For this review, take the finished solid that the model builds, in its own axes (mm). Face numbers are marked on the shaded views. A direction names the side the tool comes from. Round coordinates to 2 decimals unless told otherwise and drop trailing zeros. Write each loop counter-clockwise with the first axis right and the second up, starting at its lowest first coordinate (ties: lowest second). Pieces come first, ordered by that corner, then holes. Notation, with made-up numbers: (66.25, 49) -> (80.25, 49) arc R12 ccw to (80.25, 59) -> close; hole circle Ø11 at (-8.75, 61). An arc over 180 degrees is marked (long way). Answer in a Markdown table with one row per item.
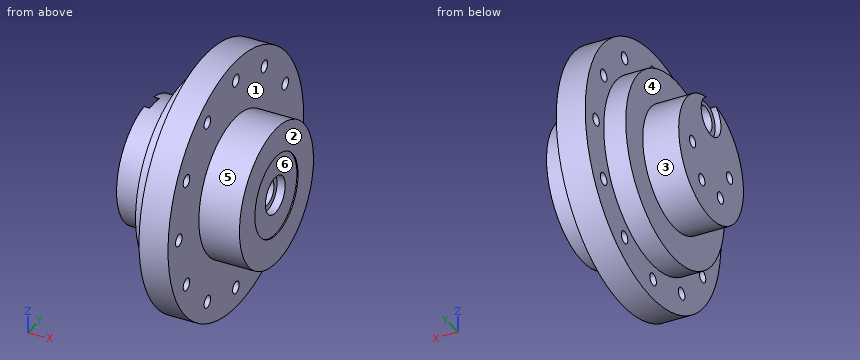
from build123d import *

# Parameters (mm, degrees)
SKETCH2_R          = 35
CUT_EXTRUDE1_DEPTH = 1
CUT_EXTRUDE2_REACH = 174.699
SKETCH3_R          = 5.25
CIRPATTERN1_COUNT  = 12
SKETCH9_R          = 5
CUT_EXTRUDE3_DEPTH = 10
CIRPATTERN2_COUNT  = 4
CIRPATTERN2_ANGLE  = 180


with BuildPart() as part:
    # Sketch1 → Revolve1 (revolve)
    with BuildSketch(Plane.XY, mode=Mode.PRIVATE) as revolve1_sk:
        Polygon((-290.135135135, 60), (-325.135135135, 60), (-325.135135135, 110), (-350.135135135, 110), (-350.135135135, 80), (-369.135135135, 80), (-369.135135135, 52.5), (-400.135135135, 52.5), (-400.135135135, 0), (-290.135135135, 0), align=None)
    revolve(revolve1_sk.sketch.rotate(Axis((-400.135135135, 0, 0), (1, 0, 0)), 90), axis=Axis((-400.135135135, 0, 0), (1, 0, 0)))

    # Sketch2 → Cut-Extrude1 (cut)
    with BuildSketch(Plane(origin=(-290.135135135, 0, 0), x_dir=(0, 0, -1), z_dir=(1, 0, 0))):
        Circle(SKETCH2_R)
    extrude(amount=-CUT_EXTRUDE1_DEPTH, mode=Mode.SUBTRACT)

    # Sketch3 → Cut-Extrude2 (cut, up to next)
    with BuildSketch(Plane(origin=(-325.135135135, 0, 0), x_dir=(0, 0, -1), z_dir=(1, 0, 0)), mode=Mode.PRIVATE) as cut_extrude2_sk1:
        with Locations((0, 92.5)):
            Circle(SKETCH3_R)
    cut_extrude2_tool1 = extrude(cut_extrude2_sk1.sketch, amount=-CUT_EXTRUDE2_REACH, mode=Mode.PRIVATE) & part.part
    cut_extrude2 = cut_extrude2_tool1.solids().sort_by_distance((-325.135135, 92.5, 0))[0]
    add(cut_extrude2, mode=Mode.SUBTRACT)

    # CirPattern1: Cut-Extrude2 ×12 about axis
    cirpattern1_axis = Axis((0, 0, 0), (1, 0, 0))
    for i in range(1, CIRPATTERN1_COUNT):
        add(cut_extrude2.rotate(cirpattern1_axis, i * 360 / CIRPATTERN1_COUNT), mode=Mode.SUBTRACT)

    # Sketch4 → Cut-Revolve1 (revolve, cut)
    with BuildSketch(Plane.XY, mode=Mode.PRIVATE) as cut_revolve1_sk:
        Polygon((-291.135135135, 16), (-298.135135135, 16), (-298.135135135, 11), (-328.635135135, 11), (-328.635135135, 17), (-353.635135135, 17), (-353.635135135, 11), (-374.135135135, 11), (-374.135135135, 16), (-381.135135135, 16), (-381.135135135, 0), (-291.135135135, 0), align=None)
    revolve(cut_revolve1_sk.sketch.rotate(Axis((-291.135135135, 0, 0), (-1, 0, 0)), 90), axis=Axis((-291.135135135, 0, 0), (-1, 0, 0)), mode=Mode.SUBTRACT)

    # Sketch8 → Cut-Revolve2 (revolve, cut)
    with BuildSketch(Plane.XY.offset(38), mode=Mode.PRIVATE) as cut_revolve2_sk:
        Polygon((-400.135135135, 0), (-313.135135135, 0), (-313.135135135, 16), (-320.135135135, 16), (-320.135135135, 11), (-332.635135135, 11), (-332.635135135, 30), (-352.635135135, 30), (-352.635135135, 11), (-395.135135135, 11), (-395.135135135, 16), (-400.135135135, 16), align=None)
    revolve(cut_revolve2_sk.sketch.rotate(Axis((-400.135135135, 0, 38), (1, 0, 0)), 90), axis=Axis((-400.135135135, 0, 38), (1, 0, 0)), mode=Mode.SUBTRACT)

    # Sketch9 → Cut-Extrude3 (cut)
    with BuildSketch(Plane.ZY.offset(400.135135135)):
        with Locations((0, 30)):
            Circle(SKETCH9_R)
    cut_extrude3 = extrude(amount=-CUT_EXTRUDE3_DEPTH, mode=Mode.SUBTRACT)

    # CirPattern2: Cut-Extrude3 ×4 about axis
    cirpattern2_axis = Axis((0, 0, 0), (-1, 0, 0))
    for i in range(1, CIRPATTERN2_COUNT):
        add(cut_extrude3.rotate(cirpattern2_axis, i * CIRPATTERN2_ANGLE / (CIRPATTERN2_COUNT - 1)), mode=Mode.SUBTRACT)


solid = part.part
1) Consider section A-A on z = 92.5. State the section outline as (x, y) points.
Solved:
| item | result |
|---|---|
| outline | (-350.14, -59.53) -> (-325.14, -59.53) -> (-325.14, -5.25) -> (-350.14, -5.25) -> close; (-350.14, 5.25) -> (-325.14, 5.25) -> (-325.14, 59.53) -> (-350.14, 59.53) -> close |
2) For line 1 (Y direction, x = -393, z = 0); line 2 (Y direction, x = -347.5, z = 0); line 3 (Z direction, x = -361, y = -4), list the stretches that pass through material, from the lowest coordinate up. Write a range as [from, to].
Solved:
| item | result |
|---|---|
| line 1 | [-52.5, -35], [-25, 25], [35, 52.5] |
| line 2 | [-110, -97.75], [-87.25, -17], [17, 87.25], [97.75, 110] |
| line 3 | [-79.9, -10.25], [10.25, 27.75], [48.25, 79.9] |
3) Consider section D-D on z = 0. State how many separate pieces and enclosed holes the cut face has, then the cut area to 3 significant figures.
Solved:
| item | result |
|---|---|
| separate pieces | 3 |
| enclosed holes | 0 |
| area | 12,800 mm² |
4) Consider section C-C on x = -309. State the section outline as (y, z) points, then the cut area to 3 significant figures.
Solved:
| item | result |
|---|---|
| outline | circle Ø120 at (0, 0); hole circle Ø22 at (0, 0) |
| area | 10,900 mm² |
5) Clearance check with flat-ended pins moving along their axes: pin 1 Ø10 at (y, z) = (82, 28.5) entering from +X; pin 2 Ø9.5 at (y, z) = (80.11, -46.25) entering from -X; pin 3 Ø10 at (y, z) = (-50.5, 79.5) entering from -X; pin 4 Ø5 at (y, z) = (-7, 71) entering from -X. State where each tip first meets the part, or that it passes through.
Solved:
| item | result |
|---|---|
| pin 1 | x = -325.14 |
| pin 2 | through |
| pin 3 | x = -350.14 |
| pin 4 | x = -369.14 |
6) Consider section B-B on y = -46.25. State the section outline as (x, z) points, then the cut area to 3 significant figures.
Solved:
| item | result |
|---|---|
| outline | (-400.14, -24.84) -> (-369.14, -24.84) -> (-369.14, -65.28) -> (-350.14, -65.28) -> (-350.14, -74.86) -> (-325.14, -74.86) -> (-325.14, -38.22) -> (-290.14, -38.22) -> (-290.14, 38.22) -> (-325.14, 38.22) -> (-325.14, 74.86) -> (-350.14, 74.86) -> (-350.14, 65.28) -> (-369.14, 65.28) -> (-369.14, 24.84) -> (-400.14, 24.84) -> close; (-350.14, -99.8) -> (-325.14, -99.8) -> (-325.14, -85.36) -> (-350.14, -85.36) -> close; (-350.14, 85.36) -> (-325.14, 85.36) -> (-325.14, 99.8) -> (-350.14, 99.8) -> close |
| area | 11,200 mm² |
7) Mouldability with a two-part tool opening along Z and no side actions: class the marked faces 4, 5 and 6 as pulls with the +Z half, pulls with the -Z half, needs draft (parallel to the pull), parting line crosses it, or undercut.
Solved:
| item | result |
|---|---|
| face 4 | needs draft |
| face 5 | parting line crosses it |
| face 6 | undercut |
8) For the marked faces 1, 2 and 3, list the 3-axis set-ups (+Z, -Z, +X, -X, +Y, -Y) from which the entire face can be reached by the end or side of a thin tool; tool diameter is ignored.
Solved:
| item | result |
|---|---|
| face 1 | +X |
| face 2 | +Z, -Z, +X, +Y, -Y |
| face 3 | -X |
